Verification items for this drawing (mm, ordinates from the low corner). Coordinates: 2 decimals unless noted, no trailing zeros. Write each loop counter-clockwise with the first axis right and the second up, starting at its lowest first coordinate (ties: lowest second). Pieces come first, ordered by that corner, then holes.
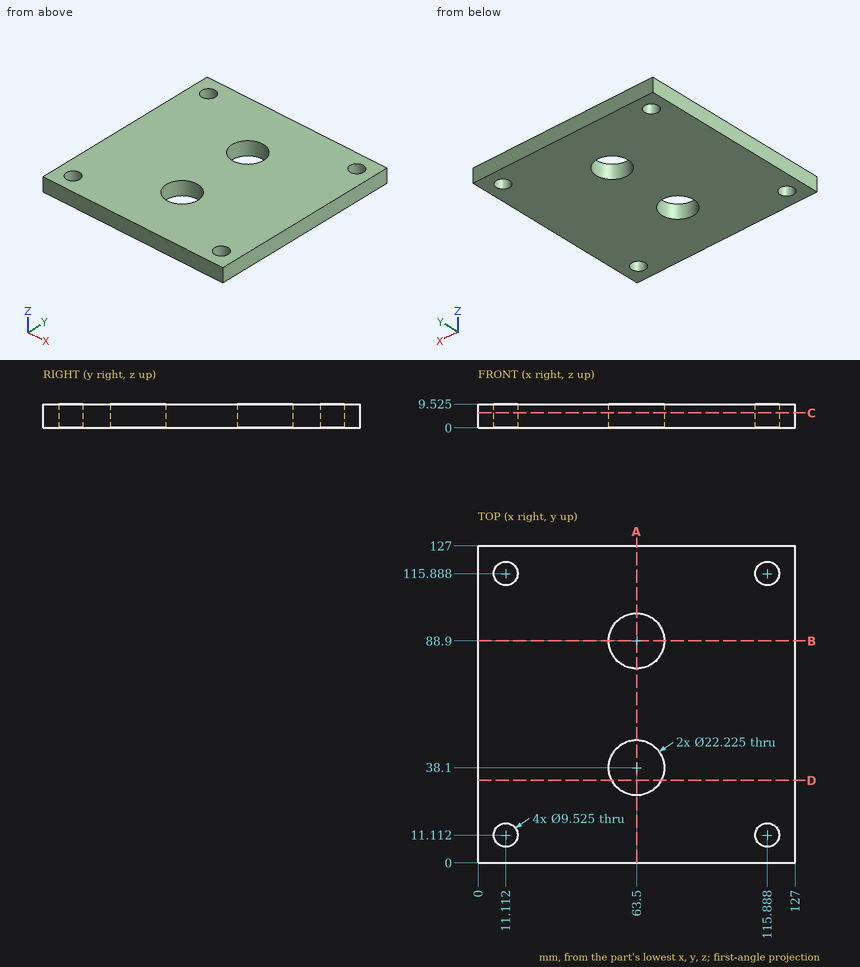
1. Sectioned sample at B-B, the plane y = 88.9. Record the boundary of the cut face in (x, z) (1 decimal).
Computed values:
outline: (0, 0) - (52.4, 0) - (52.4, 9.5) - (0, 9.5) - close; (74.6, 0) - (127, 0) - (127, 9.5) - (74.6, 9.5) - close
2. Thickness scan on line 1 along X through (y, z) = (111.5, 2) (1 decimal); line 2 along Y through (x, z) = (7, 4.5) (1 decimal); line 3 along X through (y, z) = (98.5, 7.75) (1 decimal). Record the ranges inside material, lowest first.
Computed values:
line 1: x = 0 to 9.3, 13 to 114, 117.7 to 127
line 2: y = 0 to 8.7, 13.5 to 113.5, 118.3 to 127
line 3: x = 0 to 57.9, 69.1 to 127
3. Sectioned sample at A-A, the plane x = 63.5. Record the boundary of the cut face in (y, z) (1 decimal).
Computed values:
outline: (0, 0) - (27, 0) - (27, 9.5) - (0, 9.5) - close; (49.2, 0) - (77.8, 0) - (77.8, 9.5) - (49.2, 9.5) - close; (100, 0) - (127, 0) - (127, 9.5) - (100, 9.5) - close
4. Sectioned sample at C-C, the plane z = 6. Give the number of separate pieces and of enclosed holes in the cut face, and give its area (3 significant figures).
Computed values:
separate pieces: 1
enclosed holes: 6
area: 15,100 mm2
5. Sectioned sample at D-D, the plane y = 33. Record the boundary of the cut face in (x, z) (1 decimal), and give its area (3 significant figures).
Computed values:
outline: (0, 0) - (53.6, 0) - (53.6, 9.5) - (0, 9.5) - close; (73.4, 0) - (127, 0) - (127, 9.5) - (73.4, 9.5) - close
area: 1,020 mm2
6. Gauge pin test, flat end, axial feed: pin 1 Ø11 at (x, y) = (115.89, 11.11) entering from +Z (1 decimal). Record the tip position at first contact, or that the pin passes through.
Computed values:
pin 1: stops at z = 9.5
